Input: part model. Units: mm. Frame: model coordinates. Round coordinates to 2 decimals unless told otherwise and drop trailing zeros. Order: outer loops, then holes, each group sorted by start corner. A loop starts at its lowest first (then second) coordinate and runs counter-clockwise, first axis right, second up. Notation, with made-up numbers: (-14.5, 5.5) -> (25.5, 5.5) arc R29 ccw to (25.5, 43.5) -> close; hole circle Ø5 at (37.5, 5). An arc over 180 degrees is marked (long way). Use a Markdown table: item, result.
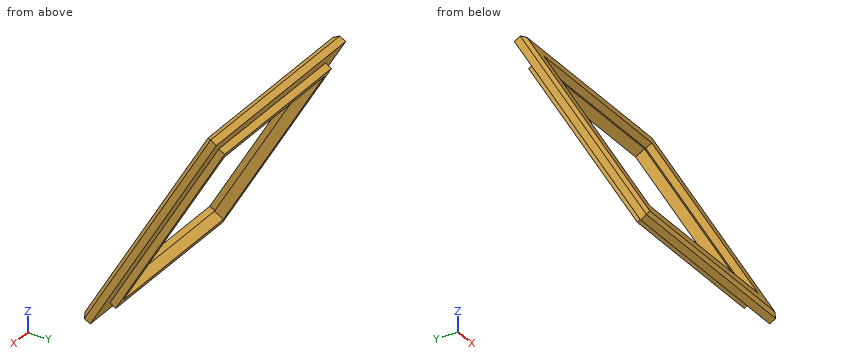
from build123d import *

# Parameters (mm, degrees)
SKETCH1_W           = 57.8
SKETCH1_H           = 74
SKETCH1_W_2         = 44.8
SKETCH1_H_2         = 59.3
BOSS_EXTRUDE1_DEPTH = 3
CHAMFER1_SIZE       = 1
SKETCH2_W           = 47.8
SKETCH2_H           = 63.8
SKETCH2_W_2         = 44.8
SKETCH2_H_2         = 59.3
BOSS_EXTRUDE2_DEPTH = 2
SKETCH4_W           = 48.2
SKETCH4_H           = 62.2
CUT_EXTRUDE1_DEPTH  = 2


with BuildPart() as part:
    # Sketch1 → Boss-Extrude1 (new body)
    with BuildSketch(Plane(origin=(0, -73.874274117, 42.651332047), x_dir=(1, 0, 0), z_dir=(0, -0.8660254037844363, 0.5000000000000041))):
        with Locations((2.02457026, 64.457304532)):
            Rectangle(SKETCH1_W, SKETCH1_H)
        with Locations((2.02457026, 64.457304532)):
            Rectangle(SKETCH1_W_2, SKETCH1_H_2, mode=Mode.SUBTRACT)
    extrude(amount=-BOSS_EXTRUDE1_DEPTH)

    # Chamfer1
    chamfer1_edges = [part.edges().sort_by_distance(p)[0] for p in [
        (-20.37542974, -41.645621851, 98.472995232),
        (2.02457026, -56.470621851, 72.795342009),
        (24.42457026, -41.645621851, 98.472995232),
        (2.02457026, -26.820621851, 124.150648454),
        (2.02457026, -23.145621851, 130.515935172),
        (30.92457026, -41.645621851, 98.472995232),
        (2.02457026, -60.145621851, 66.430055292),
        (-26.87542974, -41.645621851, 98.472995232),
    ]]
    chamfer(chamfer1_edges, length=CHAMFER1_SIZE)

    # Sketch2 → Boss-Extrude2 (add)
    with BuildSketch(Plane(origin=(0, -71.276197905, 41.151332047), x_dir=(-1, 0, 0), z_dir=(0, 0.8660254037844366, -0.5000000000000038))):
        with Locations((-2.12457026, 64.457304532)):
            Rectangle(SKETCH2_W, SKETCH2_H)
        with Locations((-2.02457026, 64.457304532)):
            Rectangle(SKETCH2_W_2, SKETCH2_H_2, mode=Mode.SUBTRACT)
    extrude(amount=BOSS_EXTRUDE2_DEPTH)

    # Sketch4 → Cut-Extrude1 (cut)
    with BuildSketch(Plane(origin=(0, -73.874274117, 42.651332047), x_dir=(1, 0, 0), z_dir=(0, -0.8660254037844366, 0.5000000000000038))):
        with Locations((2.02457026, 64.457304532)):
            Rectangle(SKETCH4_W, SKETCH4_H)
    extrude(amount=-CUT_EXTRUDE1_DEPTH, mode=Mode.SUBTRACT)


solid = part.part
1) Ray query, probe 1 along X at (y, z) = (-27.5, 120.5); probe 2 along X at (y, z) = (-43.5, 90); probe 3 along Z at (x, y) = (10, -25). Return the intervals inside material, ascending.
Answer key:
| item | result |
|---|---|
| probe 1 | x = -26.88 to -22.08, 26.12 to 30.92 |
| probe 2 | x = -26.88 to -20.38, 24.42 to 30.92 |
| probe 3 | z = 123.1 to 123.3, 124.77 to 127.3 |
2) Contact query for flat-ended pins moving along their axis: P1, Ø1.5, axis at x = -21, z = 72, coming from the -Y side; P2, Ø12, axis at x = 1, y = -54.5, coming from the -Z side; P3, Ø8, axis at x = -6.5, y = -28, coming from the -Z side; P4, Ø8, axis at x = 19.5, z = 75.5, coming from the +Y side. Output: stop coordinate, or through.
Answer key:
| item | result |
|---|---|
| P1 | stops at y = -57.36 |
| P2 | stops at z = 64.93 |
| P3 | stops at z = 122.52 |
| P4 | stops at y = -54.23 |
3) Cut plane B-B on z = 85. Return loops of the section in (x, y), and give its area (3 significant figures).
Answer key:
| item | result |
|---|---|
| outline | (-26.88, -48.27) -> (-25.88, -49.42) -> (-22.08, -49.42) -> (-22.08, -47.11) -> (-20.38, -47.11) -> (-20.38, -43.65) -> (-21.78, -43.65) -> (-21.78, -45.96) -> (-26.88, -45.96) -> close; (24.42, -47.11) -> (26.12, -47.11) -> (26.12, -49.42) -> (29.92, -49.42) -> (30.92, -48.27) -> (30.92, -45.96) -> (26.02, -45.96) -> (26.02, -43.65) -> (24.42, -43.65) -> close |
| area | 43.0 mm^2 |
4) Cut plane A-A on x = 12. Return loops of the section in (y, z).
Answer key:
| item | result |
|---|---|
| outline | (-59.65, 67.3) -> (-59.28, 65.93) -> (-57.55, 64.93) -> (-55, 69.35) -> (-53.27, 68.35) -> (-52.14, 70.3) -> (-54.74, 71.8) -> (-55.46, 70.54) -> (-57.2, 71.54) -> close; (-26.1, 125.41) -> (-24.36, 124.41) -> (-25.09, 123.15) -> (-22.49, 121.65) -> (-21.37, 123.6) -> (-23.1, 124.6) -> (-20.55, 129.02) -> (-22.28, 130.02) -> (-23.65, 129.65) -> close |
